Design review of the part built by this model. Coordinates are the model's own, in mm. A direction names the side the tool comes from. Coordinates: 2 decimals unless noted, no trailing zeros. Loops run counter-clockwise (first coordinate to the right, second up) from the corner with the lowest first, then second, coordinate; pieces in that order, holes last.
from build123d import *

# Parameters (mm, degrees)
SKETCH1_W           = 50
SKETCH1_H           = 250
BOSS_EXTRUDE1_DEPTH = 5
SKETCH2_R           = 15
CUT_EXTRUDE1_DEPTH  = 3
SKETCH5_R           = 15
CUT_EXTRUDE2_DEPTH  = 3


with BuildPart() as part:
    # Sketch1 → Boss-Extrude1 (new, symmetric)
    with BuildSketch(Plane.XY):
        Rectangle(SKETCH1_W, SKETCH1_H)
    extrude(amount=BOSS_EXTRUDE1_DEPTH, both=True)

    # Sketch2 → Cut-Extrude1 (cut)
    with BuildSketch(Plane.XY.offset(5)):
        with Locations((0, 100)):
            Circle(SKETCH2_R)
    extrude(amount=-CUT_EXTRUDE1_DEPTH, mode=Mode.SUBTRACT)

    # Sketch5 → Cut-Extrude2 (cut)
    with BuildSketch(Plane(origin=(0, 0, -5), x_dir=(-1, 0, 0), z_dir=(0, 0, -1))):
        with Locations((0, -100)):
            Circle(SKETCH5_R)
    extrude(amount=-CUT_EXTRUDE2_DEPTH, mode=Mode.SUBTRACT)


solid = part.part
Q1. The part is to be moulded in two halves that separate along Y. For faces 4 (the cylindrical face through (-3.252, 85.357, 3.521)), 5 (the flat face through (0, 2, 5)), 6 (the cylindrical face through (3.252, -114.643, -3.521)), 7 (the flat face through (0, 125, 0)), say which applies: pulls with the +Y half, pulls with the -Y half, needs draft (parallel to the pull), parting line crosses it, or undercut.
Q2. Take a section at B-B, the plane y = -100. Write out the cut boundary in (x, z), then the cut area to 3 significant figures.
Q3. Clearance check with flat-ended pins moving along their axes: pin 1 Ø15 at (x, y) = (3.5, 94) entering from +Z; pin 2 Ø15 at (x, y) = (0.5, -103) entering from -Z. State where each tip first meets the part, or that it passes through.
Q4. Take a section at D-D, the plane y = 106.5. Write out the cut boundary in (x, z), then the cut area to 3 significant figures.
Q5. For line 1 (Y direction, x = 0, z = -4.1); line 2 (X direction, y = -100.5, z = -3.25); line 3 (Y direction, x = 0, z = 3.85), list the stretches that pass through material, from the lowest coordinate up.
Q6. Take a section at A-A, the plane x = -12. Write out the cut boundary in (y, z).
Q7. Machinability: for faces 1 (the flat face through (0, -100, -2)), 2 (the flat face through (0, 2, -5)), 3 (the flat face through (0, 100, 2)), which of the approach directions +Z, -Z, +X, -X, +Y, -Y give a long, thin tool a straight path to every point of the face, cutting with its end or side? Answer none if there is none.
Q8. Take a section at C-C, the plane x = 0. Write out the cut boundary in (y, z).
Entries:
1. face 4: undercut
1. face 5: needs draft
1. face 6: undercut
1. face 7: pulls with the +Y half
2. outline: (-25, -5) - (-15, -5) - (-15, -2) - (15, -2) - (15, -5) - (25, -5) - (25, 5) - (-25, 5) - close
2. area: 410 mm2
3. pin 1: stops at z = 2
3. pin 2: stops at z = -2
4. outline: (-25, -5) - (25, -5) - (25, 5) - (13.52, 5) - (13.52, 2) - (-13.52, 2) - (-13.52, 5) - (-25, 5) - close
4. area: 419 mm2
5. line 1: y = -125 to -115, -85 to 125
5. line 2: x = -25 to -14.99, 14.99 to 25
5. line 3: y = -125 to 85, 115 to 125
6. outline: (-125, -5) - (-109, -5) - (-109, -2) - (-91, -2) - (-91, -5) - (125, -5) - (125, 5) - (109, 5) - (109, 2) - (91, 2) - (91, 5) - (-125, 5) - close
7. face 1: -Z
7. face 2: -Z, +X, -X, +Y, -Y
7. face 3: +Z
8. outline: (-125, -5) - (-115, -5) - (-115, -2) - (-85, -2) - (-85, -5) - (125, -5) - (125, 5) - (115, 5) - (115, 2) - (85, 2) - (85, 5) - (-125, 5) - close
